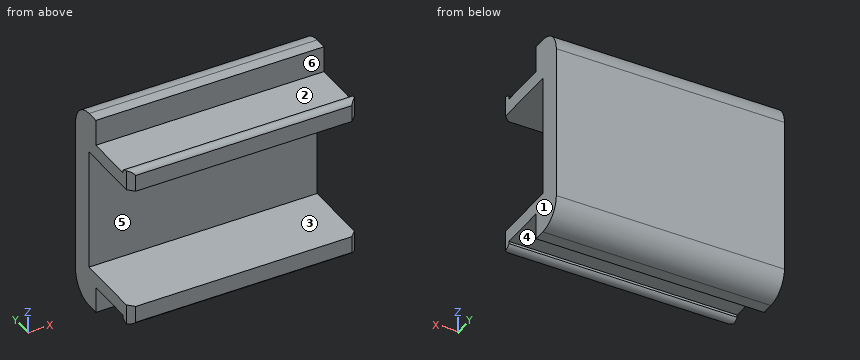
from build123d import *

# Parameters (mm, degrees)
SKETCH1_W           = 17
SKETCH1_H           = 3
BOSS_EXTRUDE1_DEPTH = 19
FILLET1_R           = 2
SKETCH2_W           = 13
SKETCH2_H           = 1
CUT_EXTRUDE1_DEPTH  = 26.670995306
SKETCH3_W           = 19
SKETCH3_H           = 0.6
BOSS_EXTRUDE2_DEPTH = 6
BOSS_EXTRUDE3_DEPTH = 19
SKETCH5_W           = 0.8
SKETCH5_H           = 6
BOSS_EXTRUDE4_DEPTH = 19
SKETCH6_W           = 0.2
SKETCH6_H           = 4
CUT_EXTRUDE11_DEPTH = 19
CHAMFER1_SIZE       = 0.5


with BuildPart() as part:
    # Sketch1 → Boss-Extrude1 (new body)
    with BuildSketch(Plane(origin=(0, 0, 0), x_dir=(0, 0, -1), z_dir=(1, 0, 0))):
        with Locations((8.5, 1.5)):
            Rectangle(SKETCH1_W, SKETCH1_H)
    extrude(amount=BOSS_EXTRUDE1_DEPTH)

    # Fillet1
    fillet1_edges = [part.edges().sort_by_distance(p)[0] for p in [
        (9.5, 3, 0),
        (9.5, 3, -17),
    ]]
    fillet(fillet1_edges, radius=FILLET1_R)

    # Sketch2 → Cut-Extrude1 (cut, through all)
    with BuildSketch(Plane(origin=(19, 0, 0), x_dir=(0, 0, -1), z_dir=(1, 0, 0))):
        with Locations((8.5, 0.5)):
            Rectangle(SKETCH2_W, SKETCH2_H)
    extrude(amount=-CUT_EXTRUDE1_DEPTH, mode=Mode.SUBTRACT)

    # Sketch3 → Boss-Extrude2 (add)
    with BuildSketch(Plane(origin=(0, 1, 0), x_dir=(-1, 0, 0), z_dir=(0, -1, 0))):
        with Locations((-9.5, 2.3)):
            Rectangle(SKETCH3_W, SKETCH3_H)
        with Locations((-9.5, 14.7)):
            Rectangle(SKETCH3_W, SKETCH3_H)
    extrude(amount=BOSS_EXTRUDE2_DEPTH)

    # Sketch4 → Boss-Extrude3 (add)
    with BuildSketch(Plane(origin=(19, 0, 0), x_dir=(0, 0, -1), z_dir=(1, 0, 0))):
        with BuildLine():
            Line((2, -5), (2, -4))
            ThreePointArc((2, -4), (1.731662479, -4.5), (2, -5))
        make_face()
        with BuildLine():
            Line((15, -5), (15, -4))
            ThreePointArc((15, -4), (15.268337521, -4.5), (15, -5))
        make_face()
    extrude(amount=-BOSS_EXTRUDE3_DEPTH)

    # Sketch5 → Boss-Extrude4 (add)
    with BuildSketch(Plane(origin=(19, 0, 0), x_dir=(0, 0, -1), z_dir=(1, 0, 0))):
        with Locations((3, -2)):
            Rectangle(SKETCH5_W, SKETCH5_H)
        with Locations((14, -2)):
            Rectangle(SKETCH5_W, SKETCH5_H)
    extrude(amount=-BOSS_EXTRUDE4_DEPTH)

    # Sketch6 → Cut-Extrude11 (cut)
    with BuildSketch(Plane(origin=(19, 0, 0), x_dir=(0, 0, -1), z_dir=(1, 0, 0))):
        with Locations((2.1, -2)):
            Rectangle(SKETCH6_W, SKETCH6_H)
        with Locations((14.9, -2)):
            Rectangle(SKETCH6_W, SKETCH6_H)
    extrude(amount=-CUT_EXTRUDE11_DEPTH, mode=Mode.SUBTRACT)

    # Chamfer1
    chamfer1_edges = [part.edges().sort_by_distance(p)[0] for p in [
        (19, -5, -2.7),
        (0, -5, -2.7),
        (0, -5, -14.3),
        (19, -5, -14.3),
    ]]
    chamfer(chamfer1_edges, length=CHAMFER1_SIZE)


solid = part.part
Source: CAD feature listing. Evaluate the final solid. Frame: model axes, mm. Face numbers are marked on the shaded views. A direction names the side the tool comes from. Coordinates: 2 decimals unless noted, no trailing zeros. Loops run counter-clockwise (first coordinate to the right, second up) from the corner with the lowest first, then second, coordinate; pieces in that order, holes last. Notation, with made-up numbers: (28.25, -13) - (51.25, -13) arc R17 ccw to (51.25, 7) - close; hole circle Ø6 at (82, -34.75). An arc over 180 degrees is marked (long way). Return JSON: item names as keys, results as strings.
Q1. Contact query for flat-ended pins moving along their axis: P1, Ø1.8, axis at x = 8, z = -1, coming from the -Y side; P2, Ø8, axis at x = 14, z = -9.5, coming from the -Y side; P3, Ø1.1, axis at x = 12.5, z = -16, coming from the -Y side. Output: stop coordinate, or through.
Results:
{"P1": "y = -4.92", "P2": "y = 1", "P3": "y = 0"}
Q2. Access query for the marked faces 4, 5 and 6. Directions: +Z, -Z, +X, -X, +Y, -Y. A direction counts if a zero-diameter tool reaches every point of the face in a straight line with its end or side. Return the directions, or none.
Results:
{"face 4": "-Z, +X, -X", "face 5": "+X, -X, -Y", "face 6": "+Z, +X, -X"}
Q3. Material intervals for line 1 along Z through (x, y) = (10, -3); line 2 along Y through (x, z) = (14, -7); line 3 along Y through (x, z) = (16.75, -1.5), sorted ascending.
Results:
{"line 1": "-14.8 to -13.6, -3.4 to -2.2", "line 2": "1 to 3", "line 3": "0 to 2.94"}
Q4. Section B-B, the plane x = 12.5. Return loops of the section in (y, z).
Results:
{"outline": "(-5, -15) arc R0.6 ccw to (-4, -15) - (-4, -14.8) - (0, -14.8) - (0, -17) - (1, -17) arc R2 ccw to (3, -15) - (3, -2) arc R2 ccw to (1, 0) - (0, 0) - (0, -2.2) - (-4, -2.2) - (-4, -2) arc R0.6 ccw to (-5, -2) - (-5, -3.4) - (1, -3.4) - (1, -13.6) - (-5, -13.6) - close"}
Q5. Section C-C, the plane y = 1.75. Return loops of the section in (x, z), plus the area to 3 significant figures.
Results:
{"outline": "(0, -16.85) - (19, -16.85) - (19, -0.15) - (0, -0.15) - close", "area": "317 mm2"}
Q6. Mould query, pull axis Z, two halves, no side actions, for the marked faces 1, 2 and 3. Classes: released by +Z, released by -Z, zero draft, split by the parting line, or undercut.
Results:
{"face 1": "zero draft", "face 2": "released by +Z", "face 3": "undercut"}
Q7. Section A-A, the plane y = -3. Return loops of the section in (x, z), plus the area to 3 significant figures.
Results:
{"outline": "(0, -14.8) - (19, -14.8) - (19, -13.6) - (0, -13.6) - close; (0, -3.4) - (19, -3.4) - (19, -2.2) - (0, -2.2) - close", "area": "45.6 mm2"}
